CAD build for the part. Positions are in the model's coordinates, mm. Round coordinates to 2 decimals unless told otherwise and drop trailing zeros. Write each loop counter-clockwise with the first axis right and the second up, starting at its lowest first coordinate (ties: lowest second). Pieces come first, ordered by that corner, then holes. Notation, with made-up numbers: (49, 22.25) - (67, 22.25) arc R15 ccw to (67, 44.25) - close; hole circle Ø11 at (-28.75, -38.5). An arc over 180 degrees is marked (long way). Use one line per item in the form item = value. Start each with the question number.
Item 1: Band-saw the part on A-A, the plane x = -202.5. List the corners of the cut face in (y, z).
Item 2: Pin check, flat tips, straight feed: pin 1 (10 mm diameter, centred on x = -80, z = 2, fed in from +Y); pin 2 (1.5 mm diameter, centred on x = -300.5, z = 2.5, fed in from +Y); pin 3 (3 mm diameter, centred on x = -41, y = 5, fed in from +Z). Stop position of each tip, or through.
Item 3: Drill centre lines: L1, parallel to X at y = -5, z = -0.5; L2, parallel to X at y = -5.25, z = -7.5; L3, parallel to X at y = -4, z = 6. Where is each one in solid material? Low to high.
from build123d import *

# Parameters (mm, degrees)
F0_R          = 4.25
F0_R_2        = 3.15
F1_DEPTH      = 442
F0_R_3        = 6.65
F2_DEPTH      = 21.5
F0_R_4        = 11
F3_DEPTH      = 28.7
F4_W          = 10.5
F4_H          = 14.3
F5_DEPTH      = 11.001
F5_DEPTH_BACK = 3.4


with BuildPart() as f1:
    # F0 (on Right) → F1 (new body)
    with BuildSketch(Plane.YZ):
        Circle(F0_R)
        Circle(F0_R_2, mode=Mode.SUBTRACT)
    extrude(amount=-F1_DEPTH)

    # F0 (on Right) → F2 (join)
    with BuildSketch(Plane.YZ):
        Circle(F0_R_3)
        Circle(F0_R, mode=Mode.SUBTRACT)
    extrude(amount=-F2_DEPTH)

    # F0 (on Right) → F3 (join)
    with BuildSketch(Plane.YZ):
        Circle(F0_R_4)
        Circle(F0_R_3, mode=Mode.SUBTRACT)
        Circle(F0_R_3)
        Circle(F0_R, mode=Mode.SUBTRACT)
        Circle(F0_R)
        Circle(F0_R_2, mode=Mode.SUBTRACT)
    extrude(amount=F3_DEPTH)

    # F4 (on Top) → F5 (cut, two sides)
    with BuildSketch(Plane.XY) as f5_sk:
        with Locations((21.65, 0)):
            Rectangle(F4_W, F4_H)
    extrude(amount=-F5_DEPTH, mode=Mode.SUBTRACT)
    extrude(f5_sk.sketch, amount=F5_DEPTH_BACK, mode=Mode.SUBTRACT)


solid = f1.part
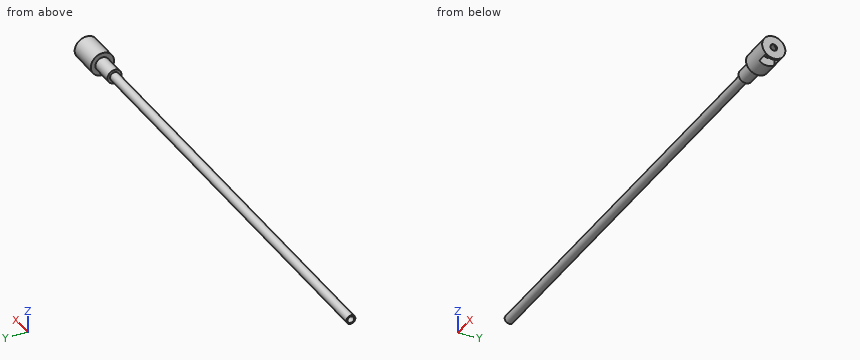
Determined:
q1.outline = circle Ø8.5 at (0, 0); hole circle Ø6.3 at (0, 0)
q2.pin_1 = 4.25
q2.pin_2 = 3.87
q2.pin_3 = 2.41
q3.L1 = -21.5 to 16.4, 26.9 to 28.7
q3.L2 = 0 to 16.4, 26.9 to 28.7
q3.L3 = 0 to 28.7
